Build history of the part. All positions in model axes, mm. Face numbers are marked on the shaded views. A direction names the side the tool comes from. Round coordinates to 2 decimals unless told otherwise and drop trailing zeros. Write each loop counter-clockwise with the first axis right and the second up, starting at its lowest first coordinate (ties: lowest second). Pieces come first, ordered by that corner, then holes. Notation, with made-up numbers: (-23.5, 47) -> (25.5, 47) arc R30 cw to (25.5, 69) -> close; hole circle Ø5 at (-4, -11.5). An arc over 180 degrees is marked (long way). One line per question, with ' | ' between items.
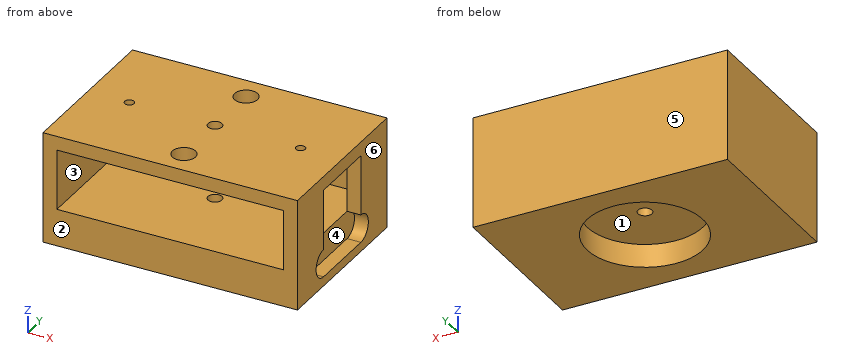
from build123d import *

# Parameters (mm, degrees)
SKETCH_W        = 55
SKETCH_H        = 36
SKETCH_R        = 1.5
PAD_DEPTH       = 24
SKETCH001_R     = 12.5
POCKET_DEPTH    = 5
SKETCH002_W     = 49
SKETCH002_H     = 13
POCKET001_DEPTH = 33
SKETCH003_R     = 1
SKETCH003_R_2   = 2.5
POCKET002_DEPTH = 3
SKETCH004_W     = 15
SKETCH004_H     = 13
POCKET003_DEPTH = 3
POCKET004_DEPTH = 3


with BuildPart() as part:
    # Sketch → Pad (new body)
    with BuildSketch(Plane.XY):
        with Locations((27.5, 18)):
            Rectangle(SKETCH_W, SKETCH_H)
        with Locations((27.5, 18)):
            Circle(SKETCH_R, mode=Mode.SUBTRACT)
    extrude(amount=PAD_DEPTH)

    # Sketch001 → Pocket (cut)
    with BuildSketch(Plane(origin=(0, 0, 0), x_dir=(1, 0, 0), z_dir=(0, 0, -1))):
        with Locations((27.5, -18)):
            Circle(SKETCH001_R)
    extrude(amount=-POCKET_DEPTH, mode=Mode.SUBTRACT)

    # Sketch002 → Pocket001 (cut)
    with BuildSketch(Plane.XZ):
        with Locations((27.5, 14.5)):
            Rectangle(SKETCH002_W, SKETCH002_H)
    extrude(amount=-POCKET001_DEPTH, mode=Mode.SUBTRACT)

    # Sketch003 → Pocket002 (cut)
    with BuildSketch(Plane.XY.offset(24)):
        with Locations((9, 18)):
            Circle(SKETCH003_R)
        with Locations((46, 18)):
            Circle(SKETCH003_R)
        with Locations((27.5, 30.5)):
            Circle(SKETCH003_R_2)
        with Locations((27.5, 5.5)):
            Circle(SKETCH003_R_2)
    extrude(amount=-POCKET002_DEPTH, mode=Mode.SUBTRACT)

    # Sketch004 → Pocket003 (cut)
    with BuildSketch(Plane.YZ.offset(55)):
        with Locations((18, 14.5)):
            Rectangle(SKETCH004_W, SKETCH004_H)
    extrude(amount=-POCKET003_DEPTH, mode=Mode.SUBTRACT)

    # Sketch005 → Pocket004 (cut)
    with BuildSketch(Plane.YZ.offset(55)):
        with BuildLine():
            ThreePointArc((10.5, 8), (7.5, 5), (10.5, 2))
            Line((10.5, 2), (25.5, 2))
            ThreePointArc((25.5, 2), (28.5, 5), (25.5, 8))
            Line((10.5, 8), (25.5, 8))
        make_face()
    extrude(amount=-POCKET004_DEPTH, mode=Mode.SUBTRACT)


solid = part.part
(1) Slice it at B-B (z = 10.5). Write the cut outline in (x, y), then the cut area to 3 significant figures.
Calculated:
outline: (0, 0) -> (3, 0) -> (3, 33) -> (52, 33) -> (52, 25.5) -> (55, 25.5) -> (55, 36) -> (0, 36) -> close; (52, 0) -> (55, 0) -> (55, 10.5) -> (52, 10.5) -> close | area: 318 mm2
(2) Slice it at A-A (x = 9). Write the cut outline in (y, z).
Calculated:
outline: (0, 0) -> (36, 0) -> (36, 24) -> (19, 24) -> (19, 21) -> (33, 21) -> (33, 8) -> (0, 8) -> close; (0, 21) -> (17, 21) -> (17, 24) -> (0, 24) -> close
(3) Wall check: line 1 (Y direction, x = 27.5, z = 22.75); line 2 (X direction, y = 18, z = 3.3); line 3 (Z direction, x = 9.5, y = 12). Give the ranges that are in metal, low to high. Write a range as from..to.
Calculated:
line 1: 0..3, 8..16.5, 19.5..28, 33..36 | line 2: 0..15, 40..52 | line 3: 0..8, 21..24
(4) Drop flat-ended pins along their axis: pin 1 (12.5 mm diameter, centred on x = 22.5, y = 14.5, fed in from -Z); pin 2 (1 mm diameter, centred on y = 9.5, z = 2.5, fed in from -X); pin 3 (4 mm diameter, centred on y = 23.5, z = 5.5, fed in from +X); pin 4 (4 mm diameter, centred on x = 27.5, y = 30.5, fed in from +Z). Give the stop position or say it passes through.
Calculated:
pin 1: z = 5 | pin 2: x = 0 | pin 3: x = 52 | pin 4: z = 8
(5) Slice it at D-D (y = 32). Write the cut outline in (x, z), then the cut area to 3 significant figures.
Calculated:
outline: (0, 0) -> (55, 0) -> (55, 24) -> (29.5, 24) -> (29.5, 21) -> (52, 21) -> (52, 8) -> (3, 8) -> (3, 21) -> (25.5, 21) -> (25.5, 24) -> (0, 24) -> close | area: 671 mm2
(6) Slice it at C-C (y = 18). State how many separate pieces and enclosed holes the cut face has, then the cut area to 3 significant figures.
Calculated:
separate pieces: 5 | enclosed holes: 0 | area: 471 mm2
(7) Mould opens along Y. For the marked faces 4, 5 and 6 say: pulls with the +Y half, pulls with the -Y half, needs draft (parallel to the pull), parting line crosses it, or undercut.
Calculated:
face 4: undercut | face 5: pulls with the +Y half | face 6: needs draft
(8) 3-axis set-ups, long thin cutter, end or side, ignore diameter. For the marked faces 1, 2 and 3: which of +Z, -Z, +X, -X, +Y, -Y reach the whole face in a straight line?
Calculated:
face 1: -Z | face 2: +Z, -Z, +X, -X, -Y | face 3: -Y
